Build history of the part. All positions in model axes, mm. A direction names the side the tool comes from. Round coordinates to 2 decimals unless told otherwise and drop trailing zeros. Use a Markdown table: item, result.
from build123d import *

# Parameters (mm, degrees)
SKETCH1_W           = 1270
SKETCH1_H           = 6.35
BOSS_EXTRUDE1_DEPTH = 152.4
SKETCH2_W           = 1270
SKETCH2_H           = 6.35
BOSS_EXTRUDE2_DEPTH = 304.8
BOSS_EXTRUDE3_DEPTH = 6.35
CUT_EXTRUDE1_DEPTH  = 1328.92833038
FILLET1_R           = 6.35
FILLET2_R           = 6.35
CUT_EXTRUDE2_DEPTH  = 775.003529142
FILLET3_R           = 12.7
FILLET4_R           = 6.35


with BuildPart() as part:
    # Sketch1 → Boss-Extrude1 (new, symmetric)
    with BuildSketch(Plane.XY):
        Rectangle(SKETCH1_W, SKETCH1_H)
    extrude(amount=BOSS_EXTRUDE1_DEPTH, both=True)

    # Sketch2 → Boss-Extrude2 (add)
    with BuildSketch(Plane(origin=(0, 3.175, 0), x_dir=(1, 0, 0), z_dir=(0, 1, 0))):
        with Locations((0, 149.225)):
            Rectangle(SKETCH2_W, SKETCH2_H)
    extrude(amount=BOSS_EXTRUDE2_DEPTH)

    # Sketch3 → Boss-Extrude3 (add)
    with BuildSketch(Plane(origin=(635, 0, 0), x_dir=(0, 0, -1), z_dir=(1, 0, 0))):
        Polygon((152.4, -3.175), (-152.4, -3.175), (-152.4, 22.225), (146.05, 307.975), (152.4, 307.975), align=None)
    boss_extrude3 = extrude(amount=BOSS_EXTRUDE3_DEPTH)

    # Mirror1: Boss-Extrude3 across plane
    add(boss_extrude3.mirror(Plane(origin=(0, 0, 0), x_dir=(0, 0, 1), z_dir=(1, 0, 0))))

    # Sketch4 → Cut-Extrude1 (cut, through all)
    with BuildSketch(Plane(origin=(641.35, 0, 0), x_dir=(0, 0, -1), z_dir=(1, 0, 0))):
        Polygon((-84.04363802, 34.925), (79.134946254, 34.925), (1.09133899, 116.437212031), align=None)
        Polygon((37.784585908, 151.569044186), (114.3, 71.652945024), (114.3, 224.82848321), align=None)
    extrude(amount=-CUT_EXTRUDE1_DEPTH, mode=Mode.SUBTRACT)

    # Fillet1
    fillet1_edges = [part.edges().sort_by_distance(p)[0] for p in [
        (638.175, 34.925, -79.134946254),
        (638.175, 34.925, 84.04363802),
        (638.175, 116.437212031, -1.09133899),
        (638.175, 71.652945024, -114.3),
        (638.175, 151.569044186, -37.784585908),
        (638.175, 224.82848321, -114.3),
    ]]
    fillet(fillet1_edges, radius=FILLET1_R)

    # Fillet2
    fillet2_edges = [part.edges().sort_by_distance(p)[0] for p in [
        (-638.175, 34.925, -79.134946254),
        (-638.175, 34.925, 84.04363802),
        (-638.175, 116.437212031, -1.09133899),
        (-638.175, 71.652945024, -114.3),
        (-638.175, 151.569044186, -37.784585908),
        (-638.175, 224.82848321, -114.3),
    ]]
    fillet(fillet2_edges, radius=FILLET2_R)

    # Sketch5 → Cut-Extrude2 (cut, through all)
    with BuildSketch(Plane(origin=(0, 0, -152.4), x_dir=(-1, 0, 0), z_dir=(0, 0, -1))):
        Polygon((-38.1, 269.875), (-498.26805665, 269.875), (-38.1, 90.65165162), align=None)
        Polygon((-104.98194335, 34.925), (-603.25, 228.987295748), (-603.25, 34.925), align=None)
        Polygon((38.1, 214.14834838), (38.1, 34.925), (498.26805665, 34.925), align=None)
        Polygon((603.25, 269.875), (104.98194335, 269.875), (603.25, 75.812704252), align=None)
    extrude(amount=-CUT_EXTRUDE2_DEPTH, mode=Mode.SUBTRACT)

    # Fillet3
    fillet3_edges = [part.edges().sort_by_distance(p)[0] for p in [
        (38.1, 90.65165162, -149.225),
        (498.26805665, 269.875, -149.225),
        (38.1, 269.875, -149.225),
        (603.25, 34.925, -149.225),
        (603.25, 228.987295748, -149.225),
        (104.98194335, 34.925, -149.225),
        (-38.1, 214.14834838, -149.225),
        (-498.26805665, 34.925, -149.225),
        (-38.1, 34.925, -149.225),
        (-104.98194335, 269.875, -149.225),
        (-603.25, 269.875, -149.225),
        (-603.25, 75.812704252, -149.225),
    ]]
    fillet(fillet3_edges, radius=FILLET3_R)

    # Fillet4
    fillet4_edges = [part.edges().sort_by_distance(p)[0] for p in [
        (0, 3.175, 152.4),
    ]]
    fillet(fillet4_edges, radius=FILLET4_R - 0.0001)  # a hair under: the kernel refuses the full size


solid = part.part
Q1. Which spindle directions (+Z, -Z, +X, -X, +Y, -Y) get a long thin tool onto all of the face, cutting with end or side? Do faces 5 (the flat face through (638.22, 185.66, -73.39)), 6 (the flat face through (374, 139.7, -149.3)), 7 (the flat face through (-9, 153, -146.05)), 8 (the flat face through (-641.35, 120, -36)). Say none if no direction does.
Response values:
| item | result |
|---|---|
| face 5 | +X, -X |
| face 6 | +Z, -Z |
| face 7 | +Z, +Y |
| face 8 | +Z, -Z, -X, +Y, -Y |
Q2. Two-plate mould, pull along Y, no slides. Class faces 1 (the flat face through (638.22, 79.42, 37.57)), 2 (the flat face through (9, -3.175, -2)), 3 (the flat face through (638.131, 163.1, 5.264)), 4 (the flat face through (635, 120, -32)): +Y half, -Y half, draft (parallel to the pull), parting line (faces both ways), or undercut.
Response values:
| item | result |
|---|---|
| face 1 | undercut |
| face 2 | -Y half |
| face 3 | +Y half |
| face 4 | draft |
Q3. Drill centre lines: L1, parallel to X at y = 187.5, z = -125; L2, parallel to Z at x = 290.5, y = 22; L3, parallel to Y at x = -568.5, z = 85.5 (3 decimals). Where is each one in solid material? Low to high.
Response values:
| item | result |
|---|---|
| L1 | x = -641.35 to -635, 635 to 641.35 |
| L2 | z = -152.4 to -146.05 |
| L3 | y = -3.175 to 3.175 |
Q4. Drop flat-ended pins along their axis: P1, Ø8, axis at x = 35.5, y = 88.5, coming from the +Z side; P2, Ø3, axis at x = -636.5, z = -23, coming from the +Y side; P3, Ø8, axis at x = -188, z = 75.5, coming from the +Y side (3 decimals); P4, Ø12, axis at y = 43, z = 45.5, coming from the +X side. Give the stop position or say it passes through.
Response values:
| item | result |
|---|---|
| P1 | stops at z = -146.05 |
| P2 | stops at y = 191.6 |
| P3 | stops at y = 3.175 |
| P4 | passes through |
Q5. Cut at B-B on z = -82. Count the separate pieces of the cut face and the enclosed holes in it, and give its area (3 significant figures).
Response values:
| item | result |
|---|---|
| separate pieces | 3 |
| enclosed holes | 0 |
| area | 10,100 mm2 |
